Geometry check sheet. Reference: the model listing, model coordinates, mm. Coordinates: 2 decimals unless noted, no trailing zeros. Write each loop counter-clockwise with the first axis right and the second up, starting at its lowest first coordinate (ties: lowest second). Pieces come first, ordered by that corner, then holes. Notation, with made-up numbers: M 31.25,28.25 L 83.25,28.25 A25 cw 83.25,62.25 Z; hole C 85.5,-31 d2. An arc over 180 degrees is marked long. Answer as a JSON object with one key per item and string values. Group by question number.
```python
from build123d import *
from OCP.BRepFilletAPI import BRepFilletAPI_MakeChamfer

# Parameters (mm, degrees)
SKETCH_1_W                   = 370
SKETCH_1_H                   = 15
EXTRUDE_1_DEPTH              = 10
SKETCH_2_R                   = 3.05
CUT_EXTRUDE_1_DEPTH          = 371.43892884
PATTERN_LINEAR_1_COUNT       = 14
PATTERN_LINEAR_1_PITCH       = 27
HOLE_WIZARD_M5_1_D           = 5.8
HOLE_WIZARD_M5_1_CBORE_D     = 10
HOLE_WIZARD_M5_1_CBORE_DEPTH = 5
CHAMFER_1_SIZE               = 1
CHAMFER_1_SIZE2              = 0.577350269


with BuildPart() as part:
    # 草图1 → 凸台-拉伸1 (new body)
    with BuildSketch(Plane.XY):
        with Locations((185, 7.5)):
            Rectangle(SKETCH_1_W, SKETCH_1_H)
    extrude(amount=EXTRUDE_1_DEPTH)

    # 草图2 → 切除-拉伸1 (cut, through all)
    with BuildSketch(Plane.XY.offset(10)):
        with Locations((8, 7.5)):
            Circle(SKETCH_2_R)
    cut_extrude_1 = extrude(amount=-CUT_EXTRUDE_1_DEPTH, mode=Mode.SUBTRACT)

    # 阵列(线性)1: 切除-拉伸1 ×14
    with Locations(*[(i * PATTERN_LINEAR_1_PITCH, 0, 0) for i in range(1, PATTERN_LINEAR_1_COUNT)]):
        add(cut_extrude_1, mode=Mode.SUBTRACT)

    # M5 六角凹头螺钉的柱形沉头孔1 (through all)
    with Locations(Plane.XY.offset(10)):
        with Locations((21, 7.5), (102, 7.5), (183, 7.5), (264, 7.5)):
            CounterBoreHole(HOLE_WIZARD_M5_1_D / 2, HOLE_WIZARD_M5_1_CBORE_D / 2, HOLE_WIZARD_M5_1_CBORE_DEPTH)

    # 倒角1: one chamfer whose edges measure the first distance from different faces: ONE call of the kernel's chamfer builder (chamfer() names one face for all edges)
    chamfer_1_edges_1 = [part.edges().sort_by_distance(p)[0] for p in [
        (4.95, 7.5, 10),
    ]]
    chamfer_1_side_1 = [part.faces().sort_by_distance(p)[0] for p in [
        (4.95, 7.5, 5),
    ]]
    chamfer_1_edges_2 = [part.edges().sort_by_distance(p)[0] for p in [
        (31.95, 7.5, 10),
    ]]
    chamfer_1_side_2 = [part.faces().sort_by_distance(p)[0] for p in [
        (31.95, 7.5, 5),
    ]]
    chamfer_1_edges_3 = [part.edges().sort_by_distance(p)[0] for p in [
        (58.95, 7.5, 10),
    ]]
    chamfer_1_side_3 = [part.faces().sort_by_distance(p)[0] for p in [
        (58.95, 7.5, 5),
    ]]
    chamfer_1_edges_4 = [part.edges().sort_by_distance(p)[0] for p in [
        (85.95, 7.5, 10),
    ]]
    chamfer_1_side_4 = [part.faces().sort_by_distance(p)[0] for p in [
        (85.95, 7.5, 5),
    ]]
    chamfer_1_edges_5 = [part.edges().sort_by_distance(p)[0] for p in [
        (112.95, 7.5, 10),
    ]]
    chamfer_1_side_5 = [part.faces().sort_by_distance(p)[0] for p in [
        (112.95, 7.5, 5),
    ]]
    chamfer_1_edges_6 = [part.edges().sort_by_distance(p)[0] for p in [
        (139.95, 7.5, 10),
    ]]
    chamfer_1_side_6 = [part.faces().sort_by_distance(p)[0] for p in [
        (139.95, 7.5, 5),
    ]]
    chamfer_1_edges_7 = [part.edges().sort_by_distance(p)[0] for p in [
        (166.95, 7.5, 10),
    ]]
    chamfer_1_side_7 = [part.faces().sort_by_distance(p)[0] for p in [
        (166.95, 7.5, 5),
    ]]
    chamfer_1_edges_8 = [part.edges().sort_by_distance(p)[0] for p in [
        (193.95, 7.5, 10),
    ]]
    chamfer_1_side_8 = [part.faces().sort_by_distance(p)[0] for p in [
        (193.95, 7.5, 5),
    ]]
    chamfer_1_edges_9 = [part.edges().sort_by_distance(p)[0] for p in [
        (220.95, 7.5, 10),
    ]]
    chamfer_1_side_9 = [part.faces().sort_by_distance(p)[0] for p in [
        (220.95, 7.5, 5),
    ]]
    chamfer_1_edges_10 = [part.edges().sort_by_distance(p)[0] for p in [
        (247.95, 7.5, 10),
    ]]
    chamfer_1_side_10 = [part.faces().sort_by_distance(p)[0] for p in [
        (247.95, 7.5, 5),
    ]]
    chamfer_1_edges_11 = [part.edges().sort_by_distance(p)[0] for p in [
        (274.95, 7.5, 10),
    ]]
    chamfer_1_side_11 = [part.faces().sort_by_distance(p)[0] for p in [
        (274.95, 7.5, 5),
    ]]
    chamfer_1_edges_12 = [part.edges().sort_by_distance(p)[0] for p in [
        (301.95, 7.5, 10),
    ]]
    chamfer_1_side_12 = [part.faces().sort_by_distance(p)[0] for p in [
        (301.95, 7.5, 5),
    ]]
    chamfer_1_edges_13 = [part.edges().sort_by_distance(p)[0] for p in [
        (328.95, 7.5, 10),
    ]]
    chamfer_1_side_13 = [part.faces().sort_by_distance(p)[0] for p in [
        (328.95, 7.5, 5),
    ]]
    chamfer_1_edges_14 = [part.edges().sort_by_distance(p)[0] for p in [
        (355.95, 7.5, 10),
    ]]
    chamfer_1_side_14 = [part.faces().sort_by_distance(p)[0] for p in [
        (355.95, 7.5, 5),
    ]]
    chamfer_1 = BRepFilletAPI_MakeChamfer(part.part.solid().wrapped)
    for e in chamfer_1_edges_1:
        chamfer_1.Add(CHAMFER_1_SIZE, CHAMFER_1_SIZE2, e.wrapped, chamfer_1_side_1[0].wrapped)  # the first distance lies on this face
    for e in chamfer_1_edges_2:
        chamfer_1.Add(CHAMFER_1_SIZE, CHAMFER_1_SIZE2, e.wrapped, chamfer_1_side_2[0].wrapped)  # the first distance lies on this face
    for e in chamfer_1_edges_3:
        chamfer_1.Add(CHAMFER_1_SIZE, CHAMFER_1_SIZE2, e.wrapped, chamfer_1_side_3[0].wrapped)  # the first distance lies on this face
    for e in chamfer_1_edges_4:
        chamfer_1.Add(CHAMFER_1_SIZE, CHAMFER_1_SIZE2, e.wrapped, chamfer_1_side_4[0].wrapped)  # the first distance lies on this face
    for e in chamfer_1_edges_5:
        chamfer_1.Add(CHAMFER_1_SIZE, CHAMFER_1_SIZE2, e.wrapped, chamfer_1_side_5[0].wrapped)  # the first distance lies on this face
    for e in chamfer_1_edges_6:
        chamfer_1.Add(CHAMFER_1_SIZE, CHAMFER_1_SIZE2, e.wrapped, chamfer_1_side_6[0].wrapped)  # the first distance lies on this face
    for e in chamfer_1_edges_7:
        chamfer_1.Add(CHAMFER_1_SIZE, CHAMFER_1_SIZE2, e.wrapped, chamfer_1_side_7[0].wrapped)  # the first distance lies on this face
    for e in chamfer_1_edges_8:
        chamfer_1.Add(CHAMFER_1_SIZE, CHAMFER_1_SIZE2, e.wrapped, chamfer_1_side_8[0].wrapped)  # the first distance lies on this face
    for e in chamfer_1_edges_9:
        chamfer_1.Add(CHAMFER_1_SIZE, CHAMFER_1_SIZE2, e.wrapped, chamfer_1_side_9[0].wrapped)  # the first distance lies on this face
    for e in chamfer_1_edges_10:
        chamfer_1.Add(CHAMFER_1_SIZE, CHAMFER_1_SIZE2, e.wrapped, chamfer_1_side_10[0].wrapped)  # the first distance lies on this face
    for e in chamfer_1_edges_11:
        chamfer_1.Add(CHAMFER_1_SIZE, CHAMFER_1_SIZE2, e.wrapped, chamfer_1_side_11[0].wrapped)  # the first distance lies on this face
    for e in chamfer_1_edges_12:
        chamfer_1.Add(CHAMFER_1_SIZE, CHAMFER_1_SIZE2, e.wrapped, chamfer_1_side_12[0].wrapped)  # the first distance lies on this face
    for e in chamfer_1_edges_13:
        chamfer_1.Add(CHAMFER_1_SIZE, CHAMFER_1_SIZE2, e.wrapped, chamfer_1_side_13[0].wrapped)  # the first distance lies on this face
    for e in chamfer_1_edges_14:
        chamfer_1.Add(CHAMFER_1_SIZE, CHAMFER_1_SIZE2, e.wrapped, chamfer_1_side_14[0].wrapped)  # the first distance lies on this face
    add(Compound.cast(chamfer_1.Shape()), mode=Mode.REPLACE)


solid = part.part
```
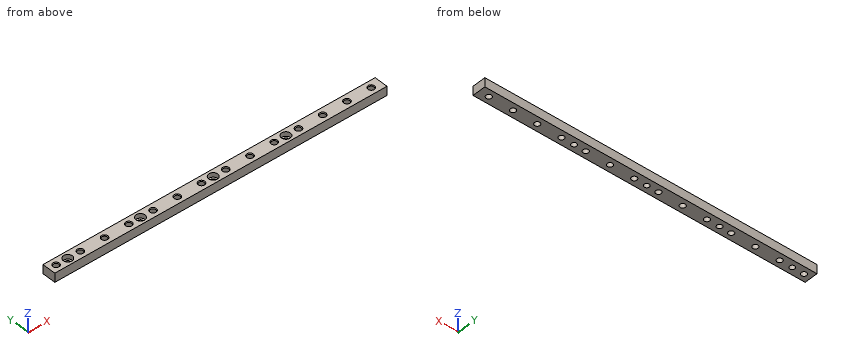
1) Section check B-B (y = 7.5). State how many separate pieces and enclosed holes the cut face has, then the cut area to 3 significant figures.
2) Go/stop test with flat-tipped pins: pin 1 Ø3.5 at (x, y) = (183, 7.5) entering from -Z; pin 2 Ø7 at (x, y) = (143, 7.5) entering from +Z. Record where each tip stops, or that it passes through.
3) Section check A-A (x = 278). Record the cut outline in (y, z).
4) Material ranges on probe 1 along Y at (x, z) = (102, 6.15); probe 2 along Y at (x, z) = (115, 7); probe 3 along Z at (x, y) = (194, 9.5), recorded low to high. Write a range as [from, to].
Entries:
{
 "1": {"separate pieces": "19", "enclosed holes": "0", "area": "2,520 mm^2"},
 "2": {"pin 1": "through", "pin 2": "z = 9.78"},
 "3": {"outline": "M 0,0 L 4.45,0 L 4.45,9 L 3.87,10 L 0,10 Z; M 10.55,0 L 15,0 L 15,10 L 11.13,10 L 10.55,9 Z"},
 "4": {"probe 1": "[0, 2.5], [12.5, 15]", "probe 2": "[0, 4.62], [10.38, 15]", "probe 3": "[0, 9.96]"}
}
